```python
from build123d import *

# Parameters (mm, degrees)
F0_R          = 10
F1_DEPTH      = 20
F2_R          = 6
F3_DEPTH      = 48
F3_DEPTH_BACK = 48
F4_W          = 50
F4_H          = 48.9827908203
F5_DEPTH      = 26


with BuildPart() as f1:
    # F0 (on Top) → F1 (new body)
    with BuildSketch(Plane.XY):
        with BuildLine():
            Line((20, -65.7692336577), (20, 65.7692336577))
            ThreePointArc((20, 65.7692336577), (0, 85.7692336577), (-20, 65.7692336577))
            Line((-20, 65.7692336577), (-20, -65.7692336577))
            ThreePointArc((-20, -65.7692336577), (0, -85.7692336577), (20, -65.7692336577))
        make_face()
        with Locations((0, -65.7692336577)):
            Circle(F0_R, mode=Mode.SUBTRACT)
        with Locations((0, 65.7692336577)):
            Circle(F0_R, mode=Mode.SUBTRACT)
    extrude(amount=F1_DEPTH)

    # F2 (on Front) → F3 (join, two sides)
    with BuildSketch(Plane.XZ) as f3_sk:
        with BuildLine():
            Line((-13, 19.118946977), (13, 19.118946977))
            Line((13, 19.118946977), (13, 30.0338421203))
            Line((13, 30.0338421203), (13, 54.118946977))
            ThreePointArc((13, 54.118946977), (0, 67.118946977), (-13, 54.118946977))
            Line((-13, 54.118946977), (-13, 30.0338421203))
            Line((-13, 30.0338421203), (-13, 19.118946977))
        make_face()
        with Locations((0, 54.118946977)):
            Circle(F2_R, mode=Mode.SUBTRACT)
    extrude(amount=F3_DEPTH)
    extrude(f3_sk.sketch, amount=-F3_DEPTH_BACK)

    # F4 (on face) → F5 (cut, through all)
    with BuildSketch(Plane.YZ.offset(13)):
        with BuildLine():
            Line((-25.0000003725, 54.118946977), (-25.0000003725, 48.1017377973))
            ThreePointArc((-25.0000003725, 48.1017377973), (-3.725e-07, 23.1017377973), (24.9999996275, 48.1017377973))
            Line((24.9999996275, 48.1017377973), (24.9999996275, 54.118946977))
            Line((24.9999996275, 54.118946977), (-25.0000003725, 54.118946977))
        make_face()
        with Locations((-3.725e-07, 78.6103423871)):
            Rectangle(F4_W, F4_H)
    extrude(amount=-F5_DEPTH, mode=Mode.SUBTRACT)


solid = f1.part
```
Here's how the part is built. I have some questions about the finished solid (model axes, mm). A direction names the side the tool comes from. Coordinates: 2 decimals unless noted, no trailing zeros. Order: outer loops, then holes, each group sorted by start corner. A loop starts at its lowest first (then second) coordinate and runs counter-clockwise, first axis right, second up.
Item 1: If we section it at D-D, the plane y = 44: List the corners of the cut face in (x, z) for me, then the cut area to 3 significant figures.
Response values:
outline: (-20, 0) - (20, 0) - (20, 20) - (13, 20) - (13, 54.12) arc R13 ccw to (-13, 54.12) - (-13, 20) - (-20, 20) - close; hole circle Ø12 at (0, 54.12)
area: 1,840 mm2
Item 2: If we section it at C-C, the plane z = 11: List the corners of the cut face in (x, y) for me, then the cut area to 3 significant figures.
Response values:
outline: (-20, -65.77) arc R20 ccw to (20, -65.77) - (20, 65.77) arc R20 ccw to (-20, 65.77) - close; hole circle Ø20 at (0, -65.77); hole circle Ø20 at (0, 65.77)
area: 5,890 mm2
Item 3: Which directions (+Z, -Z, +X, -X, +Y, -Y) give clear straight access to the entire face, cutting with the end or side of a thin tool? Please do faces 1 (the face through (13, 1, 22)), 2 (the face through (0, -48, 44)), 3 (the face through (3, 25, 60)).
Response values:
face 1: +Z, +X, +Y, -Y
face 2: +Z, +X, -X, -Y
face 3: +Z, +X, -X
Item 4: I'm going to push flat-ended pins straight in: pin 1 Ø10 at (x, z) = (-8, 42.5) entering from -Y; pin 2 Ø3 at (x, y) = (15.5, -48) entering from -Z; pin 3 Ø17 at (y, z) = (-19.5, 37.5) entering from +X; pin 4 Ø19 at (x, z) = (0, 54.12) entering from +Y. Where does each tip first touch, or does it pass through?
Response values:
pin 1: stops at y = -48
pin 2: stops at z = 0
pin 3: stops at x = 13
pin 4: stops at y = 48
Item 5: If we section it at A-A, the plane x = 0: Give the number of separate pieces and of enclosed holes in the cut face, then the cut area to 3 significant figures.
Response values:
separate pieces: 5
enclosed holes: 0
area: 4,670 mm2
Item 6: I need wall thicknesses on probe 1 along Y at (x, z) = (0, 6); probe 2 along Y at (x, z) = (4.5, 60); probe 3 along Y at (x, z) = (-5.5, 12.5). Which ranges of each line are inside material? Lowest first, please.
Response values:
probe 1: y = -85.77 to -75.77, -55.77 to 55.77, 75.77 to 85.77
probe 2: y = -48 to -25, 25 to 48
probe 3: y = -85 to -74.12, -57.42 to 57.42, 74.12 to 85
Item 7: If we section it at B-B, the plane y = -73: List the corners of the cut face in (x, z) for me, then the cut area to 3 significant figures.
Response values:
outline: (-18.65, 0) - (-6.91, 0) - (-6.91, 20) - (-18.65, 20) - close; (6.91, 0) - (18.65, 0) - (18.65, 20) - (6.91, 20) - close
area: 470 mm2
Item 8: Thinking about a two-plate mould opening in Z: for faces 4 (the face through (-1.3, -36.34, 48.26)), 5 (the face through (-14, 1, 20)), 6 (the face through (0, 48, 44)), 7 (the face through (0, 1, 0)), which applies, pulls with the +Z half, pulls with the -Z half, needs draft (parallel to the pull), parting line crosses it, or undercut?
Response values:
face 4: undercut
face 5: pulls with the +Z half
face 6: needs draft
face 7: pulls with the -Z half
